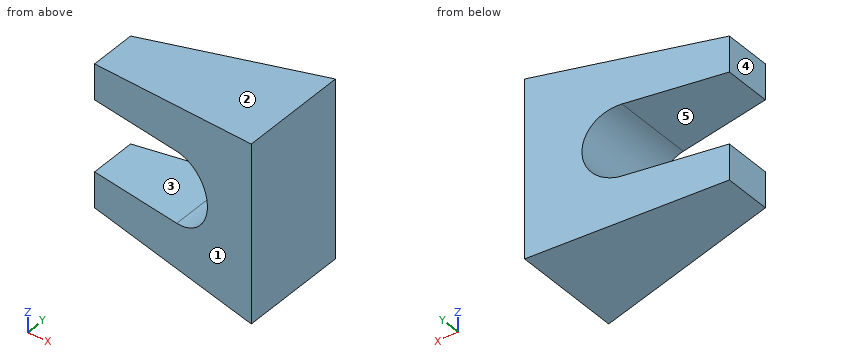
```python
from build123d import *

# Parameters (mm, degrees)
BOSS_EXTRUDE1_DEPTH     = 25
CUT_EXTRUDE1_DEPTH      = 31.731494025
CUT_EXTRUDE1_DEPTH_BACK = 31.731494025
SKETCH2_OUTSIDE_W       = 39.84
SKETCH2_OUTSIDE_H       = 64.292
CUT_EXTRUDE2_DEPTH      = 20.532560663
CUT_EXTRUDE2_DEPTH_BACK = 20.532560663


with BuildPart() as part:
    # Sketch1 → Boss-Extrude1 (new, symmetric)
    with BuildSketch(Plane(origin=(0, 0, 0), x_dir=(1, 0, 0), z_dir=(0, 1, 0))):
        Polygon((-12.773986261, -10), (-12.773986261, 10), (12.773986261, 12.5), (12.773986261, -12.5), align=None)
    extrude(amount=BOSS_EXTRUDE1_DEPTH, both=True)

    # Sketch2 outside → Cut-Extrude1 (cut, two sides: drawn at the far end of the back side and taken through both)
    with BuildSketch(Plane.XY.offset(-CUT_EXTRUDE1_DEPTH_BACK)):
        Rectangle(SKETCH2_OUTSIDE_W, SKETCH2_OUTSIDE_H)
        Polygon((-12.773986261, -3.375317421), (-12.773986261, 3.375317421), (12.773986261, 7.880114279), (12.773986261, -7.880114279), align=None, mode=Mode.SUBTRACT)
    extrude(amount=CUT_EXTRUDE1_DEPTH + CUT_EXTRUDE1_DEPTH_BACK, mode=Mode.SUBTRACT)

    # Sketch3 → Cut-Extrude2 (cut, two sides: drawn at the far end of the back side and taken through both)
    with BuildSketch(Plane(origin=(0, 0, 0), x_dir=(1, 0, 0), z_dir=(0, 1, 0)).offset(-CUT_EXTRUDE2_DEPTH_BACK)):
        with BuildLine():
            Line((-17.816892232, 5), (0.620317331, 5))
            ThreePointArc((0.620317331, 5), (5.620317331, 0), (0.620317331, -5))
            Line((0.620317331, -5), (-17.816892232, -5))
            Line((-17.816892232, -5), (-17.816892232, 5))
        make_face()
    extrude(amount=CUT_EXTRUDE2_DEPTH + CUT_EXTRUDE2_DEPTH_BACK, mode=Mode.SUBTRACT)


solid = part.part
```
Geometry: final body of the model. Coordinates: model frame, mm. Face numbers are marked on the shaded views. A direction names the side the tool comes from. Round coordinates to 2 decimals unless told otherwise and drop trailing zeros. Order: outer loops, then holes, each group sorted by start corner. A loop starts at its lowest first (then second) coordinate and runs counter-clockwise, first axis right, second up. Notation, with made-up numbers: (35, -5) -> (71, -5) arc R17 ccw to (71, 12) -> close; hole circle Ø3 at (-11.5, 31). An arc over 180 degrees is marked (long way). Write each question's results on one line, items separated by ' | '.
Q1. Section query A-A (x = -0.25). Output: boundary loops of the cut face in (y, z), and give its area (3 significant figures).
Response values:
outline: (-5.58, -11.23) -> (5.58, -11.23) -> (5.58, -5) -> (-5.58, -5) -> close; (-5.58, 5) -> (5.58, 5) -> (5.58, 11.23) -> (-5.58, 11.23) -> close | area: 139 mm²
Q2. Access query for the marked faces 4 and 5. Directions: +Z, -Z, +X, -X, +Y, -Y. A direction counts if a zero-diameter tool reaches every point of the face in a straight line with its end or side. Return the directions, or none.
Response values:
face 4: +Z, -Z, -X, +Y, -Y | face 5: -X, +Y, -Y
Q3. Section query B-B (y = 3). Output: boundary loops of the cut face in (x, z), and give its area (3 significant figures).
Response values:
outline: (-12.77, -10) -> (12.77, -12.5) -> (12.77, 12.5) -> (-12.77, 10) -> (-12.77, 5) -> (0.62, 5) arc R5 cw to (0.62, -5) -> (-12.77, -5) -> close | area: 402 mm²
Q4. Pin query (flat end, axial travel): pin 1 Ø5.5 at (x, y) = (-3.5, -1.5) entering from +Z; pin 2 Ø6 at (x, z) = (0, -5) entering from -Y; pin 3 Ø1.5 at (x, y) = (0, 3) entering from -Z. Return the tip coordinate at first contact, or that it passes through.
Response values:
pin 1: z = 11.18 | pin 2: y = -6.16 | pin 3: z = -11.32
Q5. Ray query, line 1 along Z through (x, y) = (-1.75, -0.5); line 2 along Z through (x, y) = (-0.5, 5.5); line 3 along Y through (x, z) = (11.25, -11.25). Return the intervals inside material, ascending.
Response values:
line 1: -11.08 to -5, 5 to 11.08 | line 2: -11.2 to -5, 5 to 11.2 | line 3: -7.61 to 7.61
Q6. Pull-direction query (Z, two-part tool) for the marked faces 1, 2 and 3; classes: released by +Z, released by -Z, zero draft, split by the parting line, or undercut.
Response values:
face 1: zero draft | face 2: released by +Z | face 3: undercut
Q7. Section query C-C (z = 0). Output: boundary loops of the cut face in (x, y), and give its area (3 significant figures).
Response values:
outline: (5.62, -6.62) -> (12.77, -7.88) -> (12.77, 7.88) -> (5.62, 6.62) -> close | area: 104 mm²
Q8. Section query D-D (x = -7.25). Output: boundary loops of the cut face in (y, z).
Response values:
outline: (-4.35, -10.54) -> (4.35, -10.54) -> (4.35, -5) -> (-4.35, -5) -> close; (-4.35, 5) -> (4.35, 5) -> (4.35, 10.54) -> (-4.35, 10.54) -> close
